The drawing under review shows one solid part. Ordinate dimensions are in mm from its lowest x, y, z. Coordinates: 2 decimals unless noted, no trailing zeros. Loops run counter-clockwise (first coordinate to the right, second up) from the corner with the lowest first, then second, coordinate; pieces in that order, holes last. Notation, with made-up numbers: M 30.25,60 L 56.25,60 A16 ccw 56.25,81 Z; hole C -7.75,72 d6. An arc over 180 degrees is marked long. Answer as CSV lines item,"result". Start each with the question number.
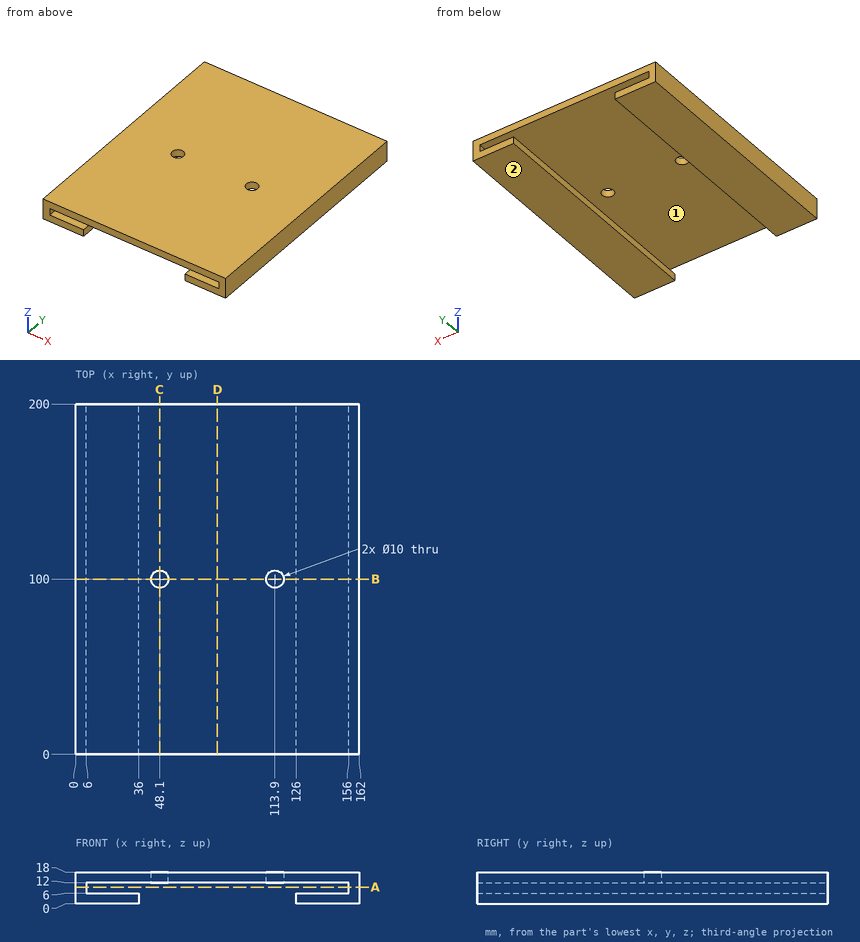
Item 1: Add section D-D (x = 81). Give the boundary of the cut face in (y, z).
Item 2: Add section A-A (z = 9.5). Give the boundary of the cut face in (x, y).
Item 3: Add section C-C (x = 48.1). Give the boundary of the cut face in (y, z).
Item 4: Mouldability with a two-part tool opening along X and no side actions: class the marked faces 1 and 2 as released by +X, released by -X, zero draft, split by the parting line, or undercut.
Item 5: Add section B-B (y = 100). Give the boundary of the cut face in (x, z), plus the area to 3 significant figures.
Item 6: For line 1 along Z through (x, y) = (8.5, 97.5); line 2 along Y through (x, z) = (113.9, 13.75); line 3 along X through (y, z) = (24, 3), list the stretches that pass through material, from the lowest coordinate up. Write a range as from..to.
Response:
1,outline,"M 0,12 L 200,12 L 200,18 L 0,18 Z"
2,outline,"M 0,0 L 6,0 L 6,200 L 0,200 Z; M 156,0 L 162,0 L 162,200 L 156,200 Z"
3,outline,"M 0,12 L 95,12 L 95,18 L 0,18 Z; M 105,12 L 200,12 L 200,18 L 105,18 Z"
4,face 1,"undercut"
4,face 2,"zero draft"
5,outline,"M 0,0 L 36,0 L 36,6 L 6,6 L 6,12 L 43.1,12 L 43.1,18 L 0,18 Z; M 53.1,12 L 108.9,12 L 108.9,18 L 53.1,18 Z; M 118.9,12 L 156,12 L 156,6 L 126,6 L 126,0 L 162,0 L 162,18 L 118.9,18 Z"
5,area,"1,360 mm²"
6,line 1,"0..6, 12..18"
6,line 2,"0..95, 105..200"
6,line 3,"0..36, 126..162"
